Check sheet for the modelled part. Datum: model origin and axes. Units: mm. A direction names the side the tool comes from. Give positions to 0.01 mm unless a question says otherwise; leave off trailing zeros. Loops run counter-clockwise (first coordinate to the right, second up) from the corner with the lowest first, then second, coordinate; pieces in that order, holes last. Notation, with made-up numbers: M 64,23.25 L 90,23.25 A35 ccw 90,55.25 Z; hole C 18,17 d7. An arc over 180 degrees is marked long. One line per question, with ' | ' between items. Start each with the question number.
from build123d import *

# Parameters (mm, degrees)
F0_R     = 6
F1_DEPTH = 8
F2_DEPTH = 2
F3_SIZE  = 3


with BuildPart() as f1:
    # F0 (on Top) → F1 (new body)
    with BuildSketch(Plane.XY):
        Circle(F0_R)
        with BuildLine():
            ThreePointArc((1, 3.614208), (2.984334, 2.270738), (3.75, 0))
            ThreePointArc((3.75, 0), (-2.270738, -2.984334), (-1, 3.614208))
            Line((-1, 3.614208), (-1, 4.75))
            Line((-1, 4.75), (1, 4.75))
            Line((1, 4.75), (1, 3.614208))
        make_face(mode=Mode.SUBTRACT)
    extrude(amount=F1_DEPTH)

    # F0 (on Top) → F2 (join)
    with BuildSketch(Plane.XY):
        with BuildLine():
            ThreePointArc((-1, 3.614208), (-2.270738, -2.984334), (3.75, 0))
            ThreePointArc((3.75, 0), (2.984334, 2.270738), (1, 3.614208))
            Line((1, 3.614208), (1, 2.75))
            Line((1, 2.75), (-1, 2.75))
            Line((-1, 2.75), (-1, 3.614208))
        make_face()
        with BuildLine():
            Line((1, 2.75), (1, 3.614208))
            ThreePointArc((1, 3.614208), (0, 3.75), (-1, 3.614208))
            Line((-1, 3.614208), (-1, 2.75))
            Line((-1, 2.75), (1, 2.75))
        make_face()
        with BuildLine():
            ThreePointArc((-1, 3.614208), (0, 3.75), (1, 3.614208))
            Line((1, 3.614208), (1, 4.75))
            Line((1, 4.75), (-1, 4.75))
            Line((-1, 4.75), (-1, 3.614208))
        make_face()
    extrude(amount=F2_DEPTH)

    # F3
    f3_edges = [f1.edges().sort_by_distance(p)[0] for p in [
        (-6, 0, 0),
    ]]
    chamfer(f3_edges, length=F3_SIZE)


solid = f1.part
Q1. Cross-section at C-C (z = 2.75). Record the cut outline in (x, y).
Q2. Cross-section at B-B (x = 0). Record the cut outline in (y, z).
Q3. Draft check along X on faces 3 (the conical face through (-0.691, -3.112, 0.188)), 4 (the flat face through (0, -4, 8)), 5 (the flat face through (1, 4, 5)). Enter one of: released by +X, released by -X, zero draft, split by the parting line, or undercut.
Q4. Access from +Z, -Z, +X, -X, +Y, -Y to the whole of each face (thin tool, end or side, straight path). Record for faces 1 (the flat face through (0, 4.75, 5)), 2 (the flat face through (0, 0, 0)).
Q5. Depth check by flat-ended pin: P1, Ø1.5, axis at x = -1.5, y = -4.5, coming from the -Z side; P2, Ø7, axis at x = 0, y = 0, coming from the +Z side; P3, Ø4, axis at x = -2.5, z = 7, coming from the -Y side. Enter the tip coordinate at first touch or a pass-through.
Q6. Material ranges on probe 1 along Y at (x, z) = (0, 4.1); probe 2 along Z at (x, y) = (-0.5, 1.75); probe 3 along Y at (x, z) = (1.25, 4.75), recorded low to high. Write a range as from..to.
Q7. Cross-section at A-A (z = 4.5). Record the cut outline in (x, y).
Solved:
1) outline: C 0,0 d11.5; hole M -1,3.61 A3.75 ccw long 1,3.61 L 1,4.75 L -1,4.75 Z
2) outline: M -6,3 L -3,0 L 3,0 L 6,3 L 6,8 L 4.75,8 L 4.75,2 L -3.75,2 L -3.75,8 L -6,8 Z
3) face 3: split by the parting line | face 4: zero draft | face 5: undercut
4) face 1: +Z | face 2: -Z, +X, -X, +Y, -Y
5) P1: stops at z = 0.99 | P2: stops at z = 2 | P3: stops at y = -5.98
6) probe 1: y = -6..-3.75, 4.75..6 | probe 2: z = 0..2 | probe 3: y = -5.87..-3.54, 3.54..5.87
7) outline: C 0,0 d12; hole M -1,3.61 A3.75 ccw long 1,3.61 L 1,4.75 L -1,4.75 Z
